```python
from build123d import *

# Parameters (mm, degrees)
EXTRUDE1_DEPTH                    = 25.4
F_10_24_TAPPED_HOLE1_D            = 3.7973
F_10_24_TAPPED_HOLE1_DEPTH        = 6.604
F_10_24_TAPPED_HOLE1_CBORE_D      = 4.826
F_10_24_TAPPED_HOLE1_CBORE_DEPTH  = 3.302
F_10_24_TAPPED_HOLE1_TIP          = 1.140824014
F_1_4_20_TAPPED_HOLE2_D           = 5.1054
F_1_4_20_TAPPED_HOLE2_DEPTH       = 16.51
F_1_4_20_TAPPED_HOLE2_CBORE_D     = 6.35
F_1_4_20_TAPPED_HOLE2_CBORE_DEPTH = 12.7
F_1_4_20_TAPPED_HOLE2_TIP         = 1.533816902


with BuildPart() as part:
    # Sketch1 → Extrude1 (new body)
    with BuildSketch(Plane.XY):
        Polygon((-6.35, 51.987941466), (6.35, 68.580838747), (6.35, -71.008376889), (-6.35, -71.008376889), align=None)
    extrude(amount=EXTRUDE1_DEPTH)

    # #10-24 Tapped Hole1
    with Locations(Plane(origin=(-37.120191611, 11.785844717, 18.061260674), x_dir=(0.6077917109691768, 0.7940964904072809, 0), z_dir=(-0.7940964904072809, 0.6077917109691768, 0))):
        with Locations((59.446155795, 5.361260674)):
            CounterBoreHole(F_10_24_TAPPED_HOLE1_D / 2, F_10_24_TAPPED_HOLE1_CBORE_D / 2, F_10_24_TAPPED_HOLE1_CBORE_DEPTH, depth=F_10_24_TAPPED_HOLE1_DEPTH)
            with Locations((0, 0, -(F_10_24_TAPPED_HOLE1_DEPTH + F_10_24_TAPPED_HOLE1_TIP / 2))):  # 118° drill point
                Cone(0, F_10_24_TAPPED_HOLE1_D / 2, F_10_24_TAPPED_HOLE1_TIP, mode=Mode.SUBTRACT)

    # 1/4-20 Tapped Hole2
    with Locations(Plane(origin=(-43.496001464, -71.008376889, 18.061260674), x_dir=(-1, 0, 0), z_dir=(0, -1, 0))):
        with Locations((-43.492926523, 5.361260674)):
            CounterBoreHole(F_1_4_20_TAPPED_HOLE2_D / 2, F_1_4_20_TAPPED_HOLE2_CBORE_D / 2, F_1_4_20_TAPPED_HOLE2_CBORE_DEPTH, depth=F_1_4_20_TAPPED_HOLE2_DEPTH)
            with Locations((0, 0, -(F_1_4_20_TAPPED_HOLE2_DEPTH + F_1_4_20_TAPPED_HOLE2_TIP / 2))):  # 118° drill point
                Cone(0, F_1_4_20_TAPPED_HOLE2_D / 2, F_1_4_20_TAPPED_HOLE2_TIP, mode=Mode.SUBTRACT)


solid = part.part
```
CAD build for the part. Positions are in the model's coordinates, mm. A direction names the side the tool comes from. Round coordinates to 2 decimals unless told otherwise and drop trailing zeros. Loops run counter-clockwise (first coordinate to the right, second up) from the corner with the lowest first, then second, coordinate; pieces in that order, holes last. Notation, with made-up numbers: (36.5, 7.25) - (93.5, 7.25) arc R13 ccw to (93.5, 21.25) - close; hole circle Ø3 at (-36, 11). An arc over 180 degrees is marked (long way). Return JSON: item names as keys, results as strings. Group by question number.
Q1. Tool access for faces 5 (the face through (2, -71.008, 10)), 6 (the face through (-0.56, -56.38, 15.19)), 7 (the face through (4.844, 54.197, 12.901)): list every direction of +Z, -Z, +X, -X, +Y, -Y with a clear straight run to the whole face (end or side of a thin tool).
Q2. Flat gauge pins, fed straight in: pin 1 Ø4 at (x, z) = (4.5, 21.5) entering from +Y; pin 2 Ø1.5 at (x, z) = (-4, 10) entering from +Y; pin 3 Ø3 at (x, z) = (0, 12.7) entering from +Y. Where does each tip first touch, or does it go through?
Q3. Band-saw the part on B-B on x = -4.5. Give the cut face in (y, z).
Q4. Band-saw the part on A-A on z = 2.5. Give the cut face in (x, y).
Q5. Two-plate mould, pull along Y, no slides. Class faces 1 (the face through (1.32, 62.01, 12.52)), 2 (the face through (-0.24, -53.23, 12.33)), 3 (the face through (4.12, 57.47, 12.62)), 4 (the face through (0, 0, 0)): +Y half, -Y half, draft (parallel to the pull), parting line (faces both ways), or undercut.
Q6. Drill centre lines: line 1 along X through (y, z) = (-56.7, 12.7); line 2 along X through (y, z) = (-62.25, 12.7); line 3 along Z through (x, y) = (-1, -65). Where is each one in solid material? Low to high. Write a range as [from, to].
Solutions:
{
 "1": {"face 5": "+Z, -Z, +X, -X, -Y", "face 6": "-Y", "face 7": "none"},
 "2": {"pin 1": "stops at y = 68.58", "pin 2": "stops at y = 56.04", "pin 3": "stops at y = 62.24"},
 "3": {"outline": "(-71.01, 0) - (54.41, 0) - (54.41, 25.4) - (-71.01, 25.4) - close"},
 "4": {"outline": "(-6.35, -71.01) - (6.35, -71.01) - (6.35, 68.58) - (-6.35, 51.99) - close"},
 "5": {"face 1": "+Y half", "face 2": "-Y half", "face 3": "undercut", "face 4": "draft"},
 "6": {"line 1": "x = [-6.35, -2.56], [2.55, 6.35]", "line 2": "x = [-6.35, -3.18], [3.17, 6.35]", "line 3": "z = [0, 9.69], [15.71, 25.4]"}
}
